```python
from build123d import *

# Parameters (mm, degrees)
BOSS_EXTRUDE1_DEPTH = 30
SKETCH2_W           = 20
SKETCH2_H           = 20
BOSS_EXTRUDE2_DEPTH = 22
SKETCH3_W           = 55
SKETCH3_H           = 35
BOSS_EXTRUDE3_DEPTH = 10


with BuildPart() as part:
    # Sketch1 → Boss-Extrude1 (new body)
    with BuildSketch(Plane(origin=(0, 0, 0), x_dir=(1, 0, 0), z_dir=(0, 1, 0))):
        Polygon((-10, 0), (-27.5, 0), (-27.5, -40), (27.5, -40), (27.5, 0), (10, 0), (10, -20), (-10, -20), align=None)
    extrude(amount=BOSS_EXTRUDE1_DEPTH)

    # Sketch2 → Boss-Extrude2 (add)
    with BuildSketch(Plane.XZ):
        with Locations((0, 10)):
            Rectangle(SKETCH2_W, SKETCH2_H)
    extrude(amount=-BOSS_EXTRUDE2_DEPTH)

    # Sketch3 → Boss-Extrude3 (add)
    with BuildSketch(Plane.XZ):
        with Locations((0, 22.5)):
            Rectangle(SKETCH3_W, SKETCH3_H)
    extrude(amount=BOSS_EXTRUDE3_DEPTH)


solid = part.part
```
Geometry check sheet. Reference: the model listing, model coordinates, mm. A direction names the side the tool comes from. Give positions to 0.01 mm unless a question says otherwise; leave off trailing zeros. Write each loop counter-clockwise with the first axis right and the second up, starting at its lowest first coordinate (ties: lowest second). Pieces come first, ordered by that corner, then holes. Notation, with made-up numbers: (-32, 6) -> (-7, 6) arc R17 cw to (-7, 38) -> close; hole circle Ø5 at (15, -10). An arc over 180 degrees is marked (long way). Use one line per item in the form item = value.
Item 1: Sectioned sample at C-C on x = 19. Enter the section's corners in (y, z), plus the area to 3 significant figures.
Results list:
outline = (-10, 5) -> (0, 5) -> (0, 0) -> (30, 0) -> (30, 40) -> (-10, 40) -> close
area = 1,550 mm2
Item 2: Mould release check, pull along X, two halves, no side actions. Record for faces 1 (the flat face through (0, 22, 10)), 2 (the flat face through (27.5, 10, 20)), 3 (the flat face through (0, 0, 3)), 4 (the flat face through (0, 26, 20)): released by +X, released by -X, zero draft, split by the parting line, or undercut.
Results list:
face_1 = undercut
face_2 = released by +X
face_3 = zero draft
face_4 = undercut
Item 3: Sectioned sample at B-B on z = 17. Enter the section's corners in (x, y), plus the area to 3 significant figures.
Results list:
outline = (-27.5, -10) -> (27.5, -10) -> (27.5, 30) -> (10, 30) -> (10, 22) -> (-10, 22) -> (-10, 30) -> (-27.5, 30) -> close
area = 2,040 mm2
Item 4: Access from +Z, -Z, +X, -X, +Y, -Y to the whole of each face (thin tool, end or side, straight path). Record for faces 5 (the flat face through (0, -5, 5)), 6 (the flat face through (-10, 26, 10)), 7 (the flat face through (0, 30, 24)).
Results list:
face_5 = -Z, +X, -X, -Y
face_6 = -Z, +Y
face_7 = +Z, -Z, +X, -X, +Y
Item 5: Depth check by flat-ended pin: pin 1 Ø4 at (x, z) = (3.5, 2.5) entering from -Y; pin 2 Ø1.5 at (x, y) = (-17.5, -2) entering from -Z; pin 3 Ø6.5 at (x, y) = (-4.5, 26) entering from -Z. Enter the tip coordinate at first touch or a pass-through.
Results list:
pin_1 = 0
pin_2 = 5
pin_3 = 20
Item 6: Scan lines: line 1 (Y direction, x = -3, z = 19); line 2 (Z direction, x = 4.5, y = -1); line 3 (X direction, y = 23, z = 11.5). Record each from-to range of solid material in increasing order.
Results list:
line_1 = -10 to 22
line_2 = 5 to 40
line_3 = -27.5 to -10, 10 to 27.5
Item 7: Sectioned sample at A-A on y = 24.5. Enter the section's corners in (x, z), plus the area to 3 significant figures.
Results list:
outline = (-27.5, 0) -> (-10, 0) -> (-10, 20) -> (10, 20) -> (10, 0) -> (27.5, 0) -> (27.5, 40) -> (-27.5, 40) -> close
area = 1,800 mm2
